Source: CAD feature listing. Evaluate the final solid. Frame: model axes, mm. A direction names the side the tool comes from. Round coordinates to 2 decimals unless told otherwise and drop trailing zeros. Write each loop counter-clockwise with the first axis right and the second up, starting at its lowest first coordinate (ties: lowest second). Pieces come first, ordered by that corner, then holes. Notation, with made-up numbers: (45, 86) -> (79, 86) arc R13 cw to (79, 100) -> close; hole circle Ø7 at (86.5, 40.5). An arc over 180 degrees is marked (long way). Put each result on its own line as item: value.
```python
from build123d import *

# Parameters (mm, degrees)
SKETCH_1_W          = 35
SKETCH_1_H          = 35
SKETCH_1_R          = 1.5
SKETCH_1_W_2        = 25
SKETCH_1_H_2        = 18
EXTRUDE_1_DEPTH     = 4
EXTRUDE_START       = -35.162864
SKETCH_3_W          = 2.5
SKETCH_3_H          = 6.077686218
EXTRUDE_2_DEPTH     = 35.162864
CUT_EXTRUDE_1_DEPTH = 35
SKETCH_5_W          = 65
SKETCH_5_H          = 72.155372437
EXTRUDE_3_DEPTH     = 5
EXTRUDE_4_DEPTH     = 35
SKETCH_7_R          = 1.5
CUT_EXTRUDE_2_DEPTH = 5


with BuildPart() as part:
    # Sketch 1 → Extrude 1 (new body)
    with BuildSketch(Plane.XY):
        with Locations((17.5, -17.5)):
            Rectangle(SKETCH_1_W, SKETCH_1_H)
        with Locations((5, -5)):
            Circle(SKETCH_1_R, mode=Mode.SUBTRACT)
        with Locations(Location((30, -30, 0), (0, 0, 180))):
            Circle(SKETCH_1_R, mode=Mode.SUBTRACT)
        with Locations((30, -5)):
            Circle(SKETCH_1_R, mode=Mode.SUBTRACT)
        with Locations(Location((5, -30, 0), (0, 0, 180))):
            Circle(SKETCH_1_R, mode=Mode.SUBTRACT)
        with Locations((17.5, -17.5)):
            Rectangle(SKETCH_1_W_2, SKETCH_1_H_2, mode=Mode.SUBTRACT)
    extrude(amount=EXTRUDE_1_DEPTH)

    # Sketch 3 → Extrude 2 (add)
    with BuildSketch(Plane(origin=(0, -33.944620864, -5.985352508), x_dir=(-1, 0, 0), z_dir=(0, -0.9848077530122076, -0.17364817766693394)).offset(EXTRUDE_START)):
        with Locations((-33.75, -3.038843109)):
            Rectangle(SKETCH_3_W, SKETCH_3_H)
        with Locations((-1.25, -3.038843109)):
            Rectangle(SKETCH_3_W, SKETCH_3_H)
    extrude(amount=EXTRUDE_2_DEPTH)

    # Sketch 4 → Cut-Extrude 1 (cut)
    with BuildSketch(Plane(origin=(35, 0, 0), x_dir=(0, 0, -1), z_dir=(1, 0, 0))):
        Polygon((-4, 0), (-6.105967267, -0.37133885), (-4, -12.314872722), align=None)
    extrude(amount=-CUT_EXTRUDE_1_DEPTH, mode=Mode.SUBTRACT)



with BuildPart() as body_2:
    # Sketch 5 → Extrude 3 (new body)
    with BuildSketch(Plane(origin=(0, -33.944620864, -5.985352508), x_dir=(-1, 0, 0), z_dir=(0, -0.9848077530122076, -0.17364817766693394))):
        with Locations((-17.5, -36.077686219)):
            Rectangle(SKETCH_5_W, SKETCH_5_H)
    extrude(amount=EXTRUDE_3_DEPTH)


with BuildPart() as part_1:
    add(part.part)

    add(body_2.part)  # Extrude 4 merges body 2
    # Sketch 6 → Extrude 4 (add)
    with BuildSketch(Plane.ZY):
        Polygon((4, -35), (4, -35.705307923), (0, -35), align=None)
    extrude(amount=-EXTRUDE_4_DEPTH)

    # Sketch 7 → Cut-Extrude 2 (cut)
    with BuildSketch(Plane(origin=(0, -33.944620864, -5.985352508), x_dir=(1, 0, 0), z_dir=(0, 0.9848077530122076, 0.17364817766693394))):
        with Locations(Location((-5, -20, 0), (0, 0, 270))):
            Circle(SKETCH_7_R)
        with Locations(Location((-5, -52.155372437, 0), (0, 0, 270))):
            Circle(SKETCH_7_R)
        with Locations(Location((40, -52.155372437, 0), (0, 0, 270))):
            Circle(SKETCH_7_R)
        with Locations(Location((40, -20, 0), (0, 0, 270))):
            Circle(SKETCH_7_R)
    extrude(amount=-CUT_EXTRUDE_2_DEPTH, mode=Mode.SUBTRACT)


solid = part_1.part
```
Q1. Cut plane B-B on y = -30. Output: boundary loops of the cut face in (x, z), and give its area (3 significant figures).
Ans:
outline: (0, -5.29) -> (2.5, -5.29) -> (2.5, 0) -> (3.5, 0) -> (3.5, 4) -> (0, 4) -> close; (6.5, 0) -> (28.5, 0) -> (28.5, 4) -> (6.5, 4) -> close; (31.5, 0) -> (32.5, 0) -> (32.5, -5.29) -> (35, -5.29) -> (35, 4) -> (31.5, 4) -> close
area: 142 mm^2
Q2. Cut plane A-A on x = 18.5. Output: boundary loops of the cut face in (y, z), and give its area (3 significant figures).
Ans:
outline: (-51.4, 64.21) -> (-38.87, -6.85) -> (-33.94, -5.99) -> (-35, 0) -> (-26.5, 0) -> (-26.5, 4) -> (-35.71, 4) -> (-46.47, 65.07) -> close; (-8.5, 0) -> (0, 0) -> (0, 4) -> (-8.5, 4) -> close
area: 430 mm^2
Q3. Draft query along Y for faces 4 (the flat face through (50, -43, 30)), 5 (the flat face through (17.71, -34.465, -3.035)), 6 (the flat face through (5, -18, 2)). Return one class per face: +Y half, -Y half, draft (parallel to the pull), parting line (faces both ways), or undercut.
Ans:
face 4: draft
face 5: +Y half
face 6: undercut
Q4. Cut plane D-D on x = 37.5. Output: boundary loops of the cut face in (y, z).
Ans:
outline: (-51.4, 64.21) -> (-38.87, -6.85) -> (-33.94, -5.99) -> (-46.47, 65.07) -> close
Q5. Cut plane C-C on y = -14. Output: boundary loops of the cut face in (x, z), and give its area (3 significant figures).
Ans:
outline: (0, -2.47) -> (2.5, -2.47) -> (2.5, 0) -> (5, 0) -> (5, 4) -> (0, 4) -> close; (30, 0) -> (32.5, 0) -> (32.5, -2.47) -> (35, -2.47) -> (35, 4) -> (30, 4) -> close
area: 52.3 mm^2
Q6. Pin query (flat end, axial travel): pin 1 (6 mm diameter, centred on x = 25, z = 54, fed in from -Y); pin 2 (4 mm diameter, centred on x = 5, y = -30, fed in from +Z); pin 3 (1.2 mm diameter, centred on x = 22.5, z = 2, fed in from +Y); pin 4 (2 mm diameter, centred on x = 9, y = -39.5, fed in from -Z). Return the tip coordinate at first contact, or that it passes through.
Ans:
pin 1: stops at y = -50.13
pin 2: stops at z = 4
pin 3: stops at y = 0
pin 4: stops at z = -6.85
Q7. Reachability of faces 1 (the flat face through (17, 0, 2)), 2 (the flat face through (30, -18, 2)), 3 (the flat face through (-15, -43, 30)) from +Z, -Z, +X, -X, +Y, -Y: full face, straight path, thin tool, end or side. Return the list, or none.
Ans:
face 1: +Z, -Z, +Y
face 2: +Z, -Z
face 3: +Z, -Z, -X, +Y, -Y
Q8. Material intervals for line 1 (X direction, y = -30, z = 3.05); line 2 (Z direction, x = 25, y = -2); line 3 (Y direction, x = 6, z = 14), sorted ascending. Write a range as [from, to].
Ans:
line 1: x = [0, 3.5], [6.5, 28.5], [31.5, 35]
line 2: z = [0, 4]
line 3: y = [-42.55, -37.47]
